from build123d import *

# Parameters (mm, degrees)
SKETCH_3_W          = 34
SKETCH_3_H          = 45
EXTRUDE_1_DEPTH     = 20
SKETCH_4_R          = 10.5
CUT_EXTRUDE_1_DEPTH = 60.841457202
SKETCH_7_W          = 15.3
SKETCH_7_H          = 12
CUT_EXTRUDE_2_DEPTH = 14
SKETCH_9_R          = 1.5
CUT_EXTRUDE_3_DEPTH = 60.841457202


with BuildPart() as part:
    # 草图3 → 凸台-拉伸1 (new body)
    with BuildSketch(Plane.XY):
        with Locations((17, 22.5)):
            Rectangle(SKETCH_3_W, SKETCH_3_H)
    extrude(amount=-EXTRUDE_1_DEPTH)

    # 草图4 → 切除-拉伸1 (cut, through all)
    with BuildSketch(Plane.XY):
        with Locations((17, 28)):
            Circle(SKETCH_4_R)
    extrude(amount=-CUT_EXTRUDE_1_DEPTH, mode=Mode.SUBTRACT)

    # 草图7 → 切除-拉伸2 (cut)
    with BuildSketch(Plane(origin=(0, 0, -20), x_dir=(-1, 0, 0), z_dir=(0, 0, -1))):
        with Locations((-17, 6)):
            Rectangle(SKETCH_7_W, SKETCH_7_H)
    extrude(amount=-CUT_EXTRUDE_2_DEPTH, mode=Mode.SUBTRACT)

    # 草图9 → 切除-拉伸3 (cut, through all)
    with BuildSketch(Plane(origin=(34, 0, 0), x_dir=(0, 0, -1), z_dir=(1, 0, 0))):
        with Locations(Location((10, 5, 0), (0, 0, 90))):
            Circle(SKETCH_9_R)
    extrude(amount=-CUT_EXTRUDE_3_DEPTH, mode=Mode.SUBTRACT)


solid = part.part
CAD build for the part. Positions are in the model's coordinates, mm. A direction names the side the tool comes from. Round coordinates to 2 decimals unless told otherwise and drop trailing zeros. Loops run counter-clockwise (first coordinate to the right, second up) from the corner with the lowest first, then second, coordinate; pieces in that order, holes last. Notation, with made-up numbers: M -19.75,63 L -2.75,63 A35 ccw -2.75,100 Z; hole C 86,59 d7. An arc over 180 degrees is marked long. One line per question, with ' | ' between items. Start each with the question number.
Item 1: Pin check, flat tips, straight feed: pin 1 Ø6 at (x, z) = (6, -10) entering from -Y; pin 2 Ø4 at (x, z) = (13.5, -15) entering from -Y. Stop position of each tip, or through.
Item 2: Cut at B-B, the plane y = 28. Write the cut outline in (x, z), plus the area to 3 significant figures.
Item 3: Wall check: line 1 (X direction, y = 6, z = -14); line 2 (Y direction, x = 17, z = -15); line 3 (Z direction, x = 4, y = 5). Give the ranges that are in metal, low to high.
Item 4: Cut at A-A, the plane z = -10. Write the cut outline in (x, y), plus the area to 3 significant figures.
Item 5: Cut at C-C, the plane x = 17. Write the cut outline in (y, z), plus the area to 3 significant figures.
Item 6: Two-plate mould, pull along Y, no slides. Class faces 1 (the cylindrical face through (4.74, 5.69, -11.33)), 2 (the flat face through (17, 12, -13)), 3 (the flat face through (17, 45, -10)), 4 (the flat face through (17, 6, -6)): pulls with the +Y half, pulls with the -Y half, needs draft (parallel to the pull), parting line crosses it, or undercut.
Item 7: Cut at D-D, the plane x = 26. Write the cut outline in (y, z), plus the area to 3 significant figures.
Item 8: Which spindle directions (+Z, -Z, +X, -X, +Y, -Y) get a long thin tool onto all of the face, cutting with end or side? Do faces 5 (the flat face through (17, 0, -5)), 6 (the flat face through (9.35, 6, -13)). Say none if no direction does.
Responses:
1) pin 1: stops at y = 0 | pin 2: stops at y = 12
2) outline: M 0,-20 L 6.5,-20 L 6.5,0 L 0,0 Z; M 27.5,-20 L 34,-20 L 34,0 L 27.5,0 Z | area: 260 mm²
3) line 1: x = 0 to 9.35, 24.65 to 34 | line 2: y = 12 to 17.5, 38.5 to 45 | line 3: z = -20 to -11.5, -8.5 to 0
4) outline: M 0,0 L 9.35,0 L 9.35,3.5 L 0,3.5 Z; M 0,6.5 L 9.35,6.5 L 9.35,12 L 24.65,12 L 24.65,6.5 L 34,6.5 L 34,45 L 0,45 Z; M 24.65,0 L 34,0 L 34,3.5 L 24.65,3.5 Z; hole C 17,28 d21 | area: 944 mm²
5) outline: M 0,-6 L 12,-6 L 12,-20 L 17.5,-20 L 17.5,0 L 0,0 Z; M 38.5,-20 L 45,-20 L 45,0 L 38.5,0 Z | area: 312 mm²
6) face 1: undercut | face 2: pulls with the -Y half | face 3: pulls with the +Y half | face 4: needs draft
7) outline: M 0,-20 L 22.59,-20 L 22.59,0 L 0,0 Z; M 33.41,-20 L 45,-20 L 45,0 L 33.41,0 Z; hole C 5,-10 d3 | area: 677 mm²
8) face 5: +Z, -Z, +X, -X, -Y | face 6: -Z, -Y
